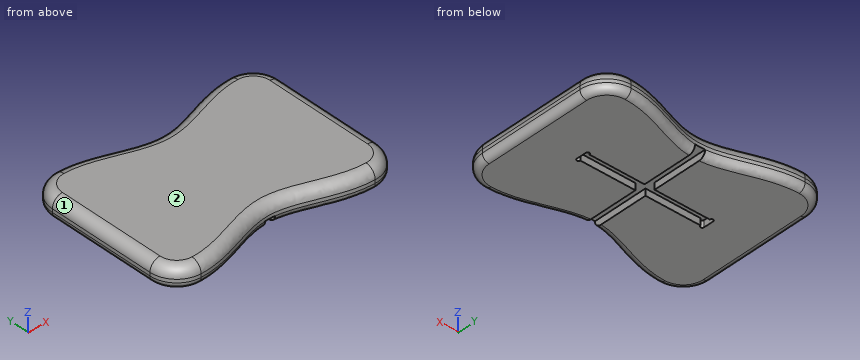
from build123d import *

# Parameters (mm, degrees)
F1_DEPTH = 38.1
F3_DEPTH = 12.7
F4_R     = 12.7
F5_R     = 19.05


with BuildPart() as f1:
    # F0 (on Top) → F1 (new body)
    with BuildSketch(Plane.XY):
        with BuildLine():
            ThreePointArc((-165.1, 152.4), (-201.021024, 137.521024), (-215.9, 101.6))
            Line((-215.9, 101.6), (-215.9, -101.6))
            ThreePointArc((-215.9, -101.6), (-201.021024, -137.521024), (-165.1, -152.4))
            add(Edge.make_bspline(
                [(-165.1, -152.4), (-101.6, -152.4), (0, -76.2), (101.6, -152.4), (165.1, -152.4)],
                knots=[0, 0, 0, 0, 169.439134, 338.878267, 338.878267, 338.878267, 338.878267], degree=3))
            ThreePointArc((165.1, -152.4), (201.021024, -137.521024), (215.9, -101.6))
            Line((215.9, -101.6), (215.9, 101.6))
            ThreePointArc((215.9, 101.6), (201.021024, 137.521024), (165.1, 152.4))
            add(Edge.make_bspline(
                [(-165.1, 152.4), (-101.6, 152.4), (0, 76.2), (101.6, 152.4), (165.1, 152.4)],
                knots=[0, 0, 0, 0, 169.439134, 338.878267, 338.878267, 338.878267, 338.878267], degree=3))
        make_face()
    extrude(amount=F1_DEPTH)

    # F2 (on face) → F3 (cut)
    with BuildSketch(Plane(origin=(0, 0, 0), x_dir=(1, 0, 0), z_dir=(0, 0, -1))):
        with BuildLine():
            ThreePointArc((-114.046, 9.525), (-117.348, 12.827), (-120.65, 9.525))
            Line((-120.65, 9.525), (-120.65, -9.525))
            ThreePointArc((-120.65, -9.525), (-117.348, -12.827), (-114.046, -9.525))
            Line((-114.046, -9.525), (-9.525, -9.525))
            Line((-9.525, -9.525), (-9.525, -114.727609))
            add(Edge.make_bspline(
                [(-9.525, -114.727609), (-6.347935, -114.448731), (0, -114.151269), (6.347935, -114.448731), (9.525, -114.727609)],
                knots=[158.852632, 158.852632, 158.852632, 158.852632, 169.439134, 180.025636, 180.025636, 180.025636, 180.025636], degree=3))
            Line((9.525, -114.727609), (9.525, -9.525))
            Line((9.525, -9.525), (114.046, -9.525))
            ThreePointArc((114.046, -9.525), (117.348, -12.827), (120.65, -9.525))
            Line((120.65, -9.525), (120.65, 9.525))
            ThreePointArc((120.65, 9.525), (117.348, 12.827), (114.046, 9.525))
            Line((114.046, 9.525), (9.525, 9.525))
            Line((9.525, 9.525), (9.525, 114.727609))
            add(Edge.make_bspline(
                [(-9.525, 114.727609), (-6.347935, 114.448731), (0, 114.151269), (6.347935, 114.448731), (9.525, 114.727609)],
                knots=[158.852632, 158.852632, 158.852632, 158.852632, 169.439134, 180.025636, 180.025636, 180.025636, 180.025636], degree=3))
            Line((-9.525, 114.727609), (-9.525, 9.525))
            Line((-9.525, 9.525), (-114.046, 9.525))
        make_face()
    extrude(amount=-F3_DEPTH, mode=Mode.SUBTRACT)

    # F4
    f4_edges = [f1.edges().sort_by_distance(p)[0] for p in [
        (-201.021024, -137.521024, 0),
        (-86.699653, -136.462181, 0),
        (86.699653, -136.462181, 0),
    ]]
    fillet(f4_edges, radius=F4_R)

    # F5
    f5_edges = [f1.edges().sort_by_distance(p)[0] for p in [
        (0, 114.3, 38.1),
    ]]
    fillet(f5_edges, radius=F5_R)


solid = f1.part
Can you work these out from the model? Positions are in its coordinate system, mm. Face numbers are marked on the shaded views. Give positions to 0.01 mm unless a question says otherwise; leave off trailing zeros. Loops run counter-clockwise (first coordinate to the right, second up) from the corner with the lowest first, then second, coordinate; pieces in that order, holes last. Notation, with made-up numbers: (51, -26) - (74, -26) arc R20 ccw to (74, -18) - close; hole circle Ø7 at (-21.75, 17). An arc over 180 degrees is marked (long way). Answer as a JSON object with one key per item and string values.
Q1. If I drill on L1, parallel to X at y = -84.5, z = 11 (3 decimals); L2, parallel to X at y = 53.5, z = 21; L3, parallel to X at y = -32.5, z = 7.5 (3 decimals), over which ranges is the centre line in solid material (lowest first)?
Geometry says:
{"L1": "-215.786 to -9.525, 9.525 to 215.786", "L2": "-215.8 to 215.8", "L3": "-214.787 to -9.525, 9.525 to 214.787"}
Q2. Imagine slicing it at A-A on y = -87. Write out the boundary of the cut face in (x, z) (3 decimals).
Geometry says:
{"outline": "(-215.9, 12.7) arc R12.7 ccw to (-203.2, 0) - (-9.525, 0) - (-9.525, 12.7) - (9.525, 12.7) - (9.525, 0) - (203.2, 0) arc R12.7 ccw to (215.9, 12.7) - (215.9, 19.05) arc R19.05 ccw to (196.85, 38.1) - (-196.85, 38.1) arc R19.05 ccw to (-215.9, 19.05) - close"}
Q3. Will these pins go through, and if not, where does the flat tip stop? P1, Ø4, axis at x = 37, z = 5, coming from the -Y side; P2, Ø10, axis at x = 46.5, z = 5.5, coming from the +Y side; P3, Ø12, axis at y = -78.5, z = 29, coming from the +X side; P4, Ø10, axis at y = -79.5, z = 8.5, coming from the +X side.
Geometry says:
{"P1": "y = -118.63", "P2": "y = 123.21", "P3": "x = 215.49", "P4": "x = 215.9"}
Q4. Imagine slicing it at B-B on y = 3. Write out the boundary of the cut face in (x, z).
Geometry says:
{"outline": "(-215.9, 12.7) arc R12.7 ccw to (-203.2, 0) - (-120.65, 0) - (-120.65, 12.7) - (120.65, 12.7) - (120.65, 0) - (203.2, 0) arc R12.7 ccw to (215.9, 12.7) - (215.9, 19.05) arc R19.05 ccw to (196.85, 38.1) - (-196.85, 38.1) arc R19.05 ccw to (-215.9, 19.05) - close"}
Q5. If we mould it in two halves opening along X, with no side actions, what happens to the marked faces 1 and 2? For each: pulls with the +X half, pulls with the -X half, needs draft (parallel to the pull), parting line crosses it, or undercut.
Geometry says:
{"face 1": "pulls with the -X half", "face 2": "needs draft"}
